Part model, mm, in its own coordinate system. Face numbers are marked on the shaded views. A direction names the side the tool comes from. Give positions to 0.01 mm unless a question says otherwise; leave off trailing zeros. Order: outer loops, then holes, each group sorted by start corner. A loop starts at its lowest first (then second) coordinate and runs counter-clockwise, first axis right, second up.
1. Slice it at D-D on z = 21. List the corners of the cut face in (x, y).
2. Drop flat-ended pins along their axis: pin 1 Ø1 at (y, z) = (-3.5, 19) entering from -X; pin 2 Ø2.5 at (x, y) = (-2.5, -3) entering from +Z; pin 3 Ø3 at (y, z) = (-1.5, 2) entering from -X. Give the stop position or say it passes through.
3. Slice it at B-B on y = -1.5. List the corners of the cut face in (x, z), and give its area (3 significant figures).
4. Mould opens along Z. For the marked faces 1, 2 and 3 say: +Z half, -Z half, draft (parallel to the pull), parting line (faces both ways), or undercut.
5. Slice it at C-C on z = 11. List the corners of the cut face in (x, y).
6. Slice it at A-A on x = 5.75. List the corners of the cut face in (y, z), and give its area (4 significant figures).
7. Which spindle directions (+Z, -Z, +X, -X, +Y, -Y) get a long thin tool onto all of the face, cutting with end or side? Do the marked faces 4, 5 and 6. Say none if no direction does.
8. Probe line 1 (Z direction, x = -3, y = -4.55); line 2 (Z direction, x = 4, y = -2.7); line 3 (X direction, y = -2.35, z = 18.5). List the from-to ranges inside material, lowest first.
Autodesk Inventor part; units mm, degrees
ref_plane "YZ Plane" through (0, 0, 0) normal (1, 0, 0) x (0, 1, 0)
ref_plane "XZ Plane" through (0, 0, 0) normal (0, 1, 0) x (-1, 0, 0)
ref_plane "XY Plane" through (0, 0, 0) normal (0, 0, 1) x (1, 0, 0)
sketch "Boceto1" plane through (0, 0, 0) normal (0, 0, 1) x (1, 0, 0)
  line L0 (0, 0) -> (15, 0)
  line L1 (15, 0) -> (15, -5)
  line L2 (15, -5) -> (0, -5)
  line L3 (0, -5) -> (0, 0)
extrude "Extrusión1" add sketch "Boceto1" along normal blind 40
sketch "Boceto2" plane through (0, 0, 0) normal (0, 1, 0) x (1, 0, 0)
  line L0 (0, -40) -> (15, -40)
  line L1 (6.174, -21.75) -> (6.174, -18.25)
  line L2 (2.774, -22.75) -> (5.174, -22.75)
  line L3 (5.174, -17.25) -> (2.774, -17.25)
  line L4 (6.174, -18.25) -> (5.174, -18.25)
  line L5 (2.774, -18.25) -> (0, -18.25)
  line L6 (2.774, -17.25) -> (2.774, -18.25)
  line L7 (2.774, -21.75) -> (2.774, -22.75)
  line L8 (5.174, -22.75) -> (5.174, -21.75)
  line L9 (5.174, -18.25) -> (5.174, -17.25)
  line L10 (0, -21.75) -> (2.774, -21.75)
  line L11 (5.174, -21.75) -> (6.174, -21.75)
  line L12 (0, -10) -> (-5, -10)
  line L13 (-5, -10) -> (-5, -4)
  line L14 (-5, -4) -> (0, -4)
  line L15 (0, -4) -> (0, -10)
  line L16 (0, -36) -> (-5, -36)
  line L17 (-5, -36) -> (-5, -30)
  line L18 (-5, -30) -> (0, -30)
  line L19 (0, -30) -> (0, -36)
  line L20 (0, 0) -> (0, -40)
  dimension "d7" = 3.5
  dimension "d8" = 2.4
  dimension "d12" = 18.25
  dimension "d14" = 6
  dimension "d15" = 5
  dimension "d16" = 5
  dimension "d17" = 6
  dimension "d18" = 4
  dimension "d19" = 20
extrude "Extrusión3" cut sketch "Boceto2" against normal through all
sketch "Boceto3" plane through (0, 0, 0) normal (0, 1, 0) x (1, 0, 0)
  line L0 (2.774, -21.75) -> (0, -21.75)
  line L1 (0, -18.25) -> (2.774, -18.25)
  line L2 (-5, -10) -> (-5, -4)
  line L3 (-5, -36) -> (-5, -30)
  line L4 (-5, -36) -> (0, -36)
  line L5 (-5, -30) -> (0, -30)
  line L6 (-5, -4) -> (0, -4)
  line L7 (-5, -10) -> (0, -10)
  line L8 (0, -4) -> (0, -10)
  line L9 (0, -30) -> (0, -36)
extrude "Extrusión4" add sketch "Boceto3" against normal blind 5
sketch "Boceto4" plane through (15, -5, 0) normal (1, 0, 0) x (0, 0, -1)
  arc A0 (-37.4947, 0.496) -> (-38.4947, 0.496) centre (-37.9947, 0.496) ccw
  line L0 (-38.4947, 0.496) -> (-38.4947, -0.004)
  line L1 (-37.4947, 0.496) -> (-37.4947, -0.004)
  line L2 (-39.4947, 0.496) -> (-39.4947, -0.004)
  arc A1 (-39.4947, 0.496) -> (-39.9947, 0.996) centre (-39.9947, 0.496) ccw
  arc A2 (-35.9947, 0.996) -> (-36.4947, 0.496) centre (-35.9947, 0.496) ccw
  line L3 (-36.4947, -0.004) -> (-36.4947, 0.496)
  arc A3 (-33.4947, 0.496) -> (-34.4947, 0.496) centre (-33.9947, 0.496) ccw
  line L4 (-34.4947, 0.496) -> (-34.4947, -0.004)
  line L5 (-33.4947, 0.496) -> (-33.4947, -0.004)
  line L6 (-35.4947, 0.496) -> (-35.4947, -0.004)
  arc A4 (-35.4947, 0.496) -> (-35.9947, 0.996) centre (-35.9947, 0.496) ccw
  arc A5 (-31.9947, 0.996) -> (-32.4947, 0.496) centre (-31.9947, 0.496) ccw
  line L7 (-32.4947, -0.004) -> (-32.4947, 0.496)
  arc A6 (-29.4947, 0.496) -> (-30.4947, 0.496) centre (-29.9947, 0.496) ccw
  line L8 (-30.4947, 0.496) -> (-30.4947, -0.004)
  line L9 (-29.4947, 0.496) -> (-29.4947, -0.004)
  line L10 (-31.4947, 0.496) -> (-31.4947, -0.004)
  arc A7 (-31.4947, 0.496) -> (-31.9947, 0.996) centre (-31.9947, 0.496) ccw
  arc A8 (-27.9947, 0.996) -> (-28.4947, 0.496) centre (-27.9947, 0.496) ccw
  line L11 (-28.4947, -0.004) -> (-28.4947, 0.496)
  line L12 (-26.4947, 0.496) -> (-26.4947, -0.004)
  line L13 (-25.4947, 0.496) -> (-25.4947, -0.004)
  line L14 (-27.4947, 0.496) -> (-27.4947, -0.004)
  line L15 (-24.4947, -0.004) -> (-24.4947, 0.496)
  arc A9 (-23.9947, 0.996) -> (-24.4947, 0.496) centre (-23.9947, 0.496) ccw
  arc A10 (-25.4947, 0.496) -> (-26.4947, 0.496) centre (-25.9947, 0.496) ccw
  arc A11 (-27.4947, 0.496) -> (-27.9947, 0.996) centre (-27.9947, 0.496) ccw
  arc A12 (-21.4947, 0.496) -> (-22.4947, 0.496) centre (-21.9947, 0.496) ccw
  line L16 (-22.4947, 0.496) -> (-22.4947, -0.004)
  line L17 (-21.4947, 0.496) -> (-21.4947, -0.004)
  line L18 (-23.4947, 0.496) -> (-23.4947, -0.004)
  arc A13 (-23.4947, 0.496) -> (-23.9947, 0.996) centre (-23.9947, 0.496) ccw
  arc A14 (-19.9947, 0.996) -> (-20.4947, 0.496) centre (-19.9947, 0.496) ccw
  line L19 (-20.4947, -0.004) -> (-20.4947, 0.496)
  line L20 (-18.4947, 0.496) -> (-18.4947, -0.004)
  line L21 (-17.4947, 0.496) -> (-17.4947, -0.004)
  line L22 (-19.4947, 0.496) -> (-19.4947, -0.004)
  line L23 (-16.4947, -0.004) -> (-16.4947, 0.496)
  arc A15 (-15.9947, 0.996) -> (-16.4947, 0.496) centre (-15.9947, 0.496) ccw
  arc A16 (-17.4947, 0.496) -> (-18.4947, 0.496) centre (-17.9947, 0.496) ccw
  arc A17 (-19.4947, 0.496) -> (-19.9947, 0.996) centre (-19.9947, 0.496) ccw
  arc A18 (-15.4947, 0.496) -> (-15.9947, 0.996) centre (-15.9947, 0.496) ccw
  line L24 (-14.4947, 0.496) -> (-14.4947, -0.004)
  arc A19 (-13.4947, 0.496) -> (-14.4947, 0.496) centre (-13.9947, 0.496) ccw
  line L25 (-13.4947, 0.496) -> (-13.4947, -0.004)
  line L26 (-12.4947, -0.004) -> (-12.4947, 0.496)
  arc A20 (-11.9947, 0.996) -> (-12.4947, 0.496) centre (-11.9947, 0.496) ccw
  arc A21 (-11.4947, 0.496) -> (-11.9947, 0.996) centre (-11.9947, 0.496) ccw
  line L27 (-11.4947, 0.496) -> (-11.4947, -0.004)
  line L28 (-15.4947, 0.496) -> (-15.4947, -0.004)
  line L29 (-10.4947, 0.496) -> (-10.4947, -0.004)
  arc A22 (-9.4947, 0.496) -> (-10.4947, 0.496) centre (-9.9947, 0.496) ccw
  line L30 (-9.4947, 0.496) -> (-9.4947, -0.004)
  line L31 (-8.4947, -0.004) -> (-8.4947, 0.496)
  arc A23 (-7.9947, 0.996) -> (-8.4947, 0.496) centre (-7.9947, 0.496) ccw
  arc A24 (0.0053, 0.996) -> (-0.4947, 0.496) centre (0.0053, 0.496) ccw
  line L32 (-0.4947, -0.004) -> (-0.4947, 0.496)
  arc A25 (-5.4947, 0.496) -> (-6.4947, 0.496) centre (-5.9947, 0.496) ccw
  line L33 (-6.4947, 0.496) -> (-6.4947, -0.004)
  line L34 (-7.4947, 0.496) -> (-7.4947, -0.004)
  arc A26 (-7.4947, 0.496) -> (-7.9947, 0.996) centre (-7.9947, 0.496) ccw
  line L35 (-5.4947, 0.496) -> (-5.4947, -0.004)
  line L36 (-4.4947, -0.004) -> (-4.4947, 0.496)
  arc A27 (-3.9947, 0.996) -> (-4.4947, 0.496) centre (-3.9947, 0.496) ccw
  arc A28 (-3.4947, 0.496) -> (-3.9947, 0.996) centre (-3.9947, 0.496) ccw
  line L37 (-3.4947, 0.496) -> (-3.4947, -0.004)
  line L38 (-2.4947, 0.496) -> (-2.4947, -0.004)
  arc A29 (-1.4947, 0.496) -> (-2.4947, 0.496) centre (-1.9947, 0.496) ccw
  line L39 (-1.4947, 0.496) -> (-1.4947, -0.004)
  line L40 (-0.4947, -0.004) -> (0.0053, -0.004)
  line L41 (-2.4947, -0.004) -> (-1.4947, -0.004)
  line L42 (-4.4947, -0.004) -> (-3.4947, -0.004)
  line L43 (-6.4947, -0.004) -> (-5.4947, -0.004)
  line L44 (-8.4947, -0.004) -> (-7.4947, -0.004)
  line L45 (-10.4947, -0.004) -> (-9.4947, -0.004)
  line L46 (-12.4947, -0.004) -> (-11.4947, -0.004)
  line L47 (-14.4947, -0.004) -> (-13.4947, -0.004)
  line L48 (-16.4947, -0.004) -> (-15.4947, -0.004)
  line L49 (-18.4947, -0.004) -> (-17.4947, -0.004)
  line L50 (-24.4947, -0.004) -> (-23.4947, -0.004)
  line L51 (-22.4947, -0.004) -> (-21.4947, -0.004)
  line L52 (-20.4947, -0.004) -> (-19.4947, -0.004)
  line L53 (-26.4947, -0.004) -> (-25.4947, -0.004)
  line L54 (-28.4947, -0.004) -> (-27.4947, -0.004)
  line L55 (-30.4947, -0.004) -> (-29.4947, -0.004)
  line L56 (-32.4947, -0.004) -> (-31.4947, -0.004)
  line L57 (-34.4947, -0.004) -> (-33.4947, -0.004)
  line L58 (-36.4947, -0.004) -> (-35.4947, -0.004)
  line L59 (-39.9947, -0.004) -> (-39.4947, -0.004)
  line L60 (-38.4947, -0.004) -> (-37.4947, -0.004)
  line L61 (0.0053, -0.004) -> (0.0053, 0.996)
  line L62 (-39.9947, -0.004) -> (-40.0154, -0.004)
  line L63 (-40.0154, -0.004) -> (-40.0154, 0.996)
  line L64 (-40.0154, 0.996) -> (-39.9947, 0.996)
  point P0 (-32.9947, 0.496)
  point P1 (-30.9947, 0.496)
  point P2 (-28.9947, 0.496)
  point P3 (-24.9947, 0.496)
  point P4 (-26.9947, 0.496)
  point P5 (-22.9947, 0.496)
  point P6 (-20.9947, 0.496)
  point P7 (-16.9947, 0.496)
  point P8 (-18.9947, 0.496)
  point P9 (-10.9947, 0.496)
  point P10 (-8.9947, 0.496)
  point P11 (-12.9947, 0.496)
  point P12 (-14.9947, 0.496)
  point P13 (-2.9947, 0.496)
  point P14 (-0.9947, 0.496)
  point P15 (-4.9947, 0.496)
  point P16 (-6.9947, 0.496)
  dimension "d49" = 4
  dimension "d50" = 8
  dimension "d51" = 4
extrude "Extrusión5" cut sketch "Boceto4" against normal blind 8
properties part number "brida correas eje y"
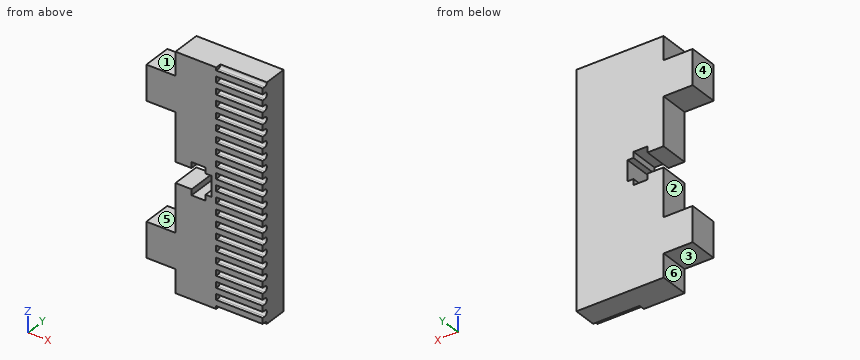
Data:
1. outline: (6.17, -5) - (15, -5) - (15, 0) - (6.17, 0) - close
2. pin 1: stops at x = 6.17
2. pin 2: stops at z = 36
2. pin 3: stops at x = 0
3. outline: (-5, 4) - (0, 4) - (0, 0) - (15, 0) - (15, 40) - (0, 40) - (0, 36) - (-5, 36) - (-5, 30) - (0, 30) - (0, 21.75) - (2.77, 21.75) - (2.77, 22.75) - (5.17, 22.75) - (5.17, 21.75) - (6.17, 21.75) - (6.17, 18.25) - (5.17, 18.25) - (5.17, 17.25) - (2.77, 17.25) - (2.77, 18.25) - (0, 18.25) - (0, 10) - (-5, 10) - close
3. area: 634 mm2
4. face 1: +Z half
4. face 2: undercut
4. face 3: -Z half
5. outline: (0, -5) - (15, -5) - (15, 0) - (0, 0) - close
6. outline: (-5, 0) - (0, 0) - (0, 18.25) - (-5, 18.25) - close; (-5, 21.75) - (0, 21.75) - (0, 40) - (-5, 40) - close
6. area: 182.5 mm2
7. face 4: +Z, -Z, -X, +Y, -Y
7. face 5: -X, +Y, -Y
7. face 6: -Z, -X, +Y, -Y
8. line 1: z = 4 to 10, 30 to 36
8. line 2: z = 0 to 17.25, 22.75 to 40
8. line 3: x = 6.17 to 15
